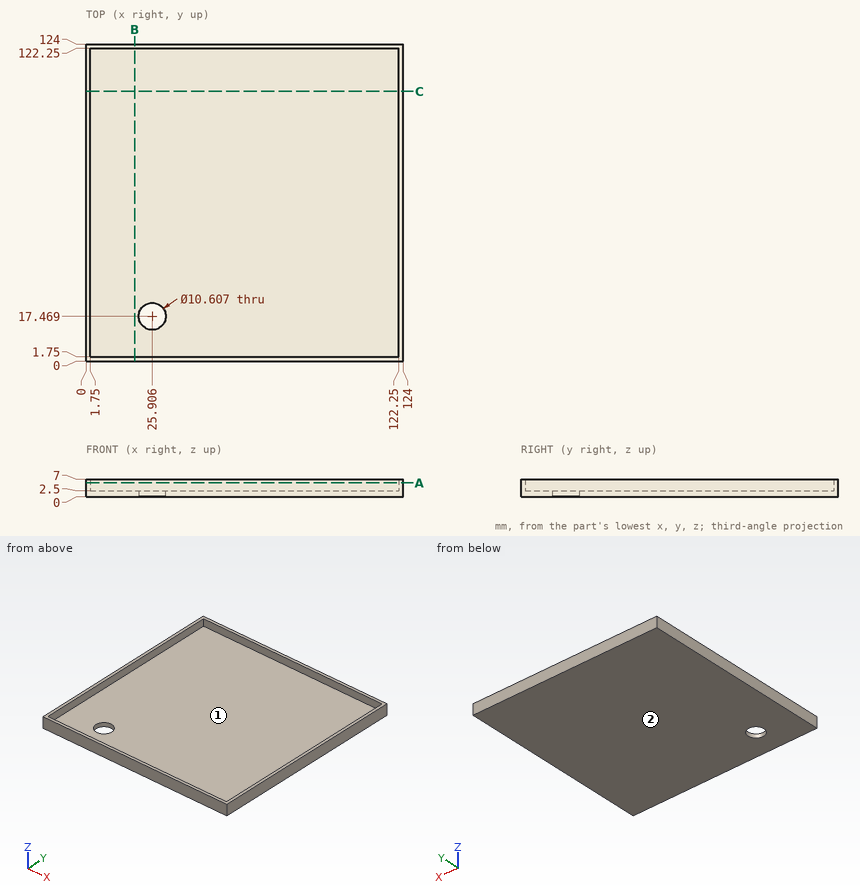
The figure shows three views and two pictorial views of one solid part (mm, origin at its lowest corner). Answer the questions. A direction names the side the tool comes from. Give positions to 0.01 mm unless a question says otherwise; leave off trailing zeros. Write each loop counter-clockwise with the first axis right and the second up, starting at its lowest first coordinate (ties: lowest second). Pieces come first, ordered by that corner, then holes.
Q1. A tool of negligible diameter and unlimited length cuts with its end or side. For the marked faces 1 and 2, from which of +Z, -Z, +X, -X, +Y, -Y can it reach the whole face along a straight path? Write none if from no direction.
Answer:
face 1: +Z
face 2: -Z, +X, -X, +Y, -Y
Q2. The part is cut by section A-A on z = 5.5. Give the vertices of the cut face in (x, y).
Answer:
outline: (0, 0) - (124, 0) - (124, 124) - (0, 124) - close; hole (1.75, 1.75) - (122.25, 1.75) - (122.25, 122.25) - (1.75, 122.25) - close
Q3. Given pin 1 (10 mm diameter, centred on x = 61, y = 19.5, fed in from +Z), flat-ended and moving along its own axis, determine where the tip first touches the part or whether it passes through.
Answer:
pin 1: stops at z = 2.5
Q4. The part is cut by section B-B on x = 19. Give the vertices of the cut face in (y, z), and give its area (3 significant figures).
Answer:
outline: (0, 0) - (124, 0) - (124, 7) - (122.25, 7) - (122.25, 2.5) - (1.75, 2.5) - (1.75, 7) - (0, 7) - close
area: 326 mm2
Q5. Straight lines are drawn through the part: L1, parallel to X at y = 48, z = 4; L2, parallel to Z at x = 13, y = 71.5. For each, find the intervals that lie inside material, in ascending order.
Answer:
L1: x = 0 to 1.75, 122.25 to 124
L2: z = 0 to 2.5
